The model under review builds one solid part; all positions refer to its coordinate system, in mm. A direction names the side the tool comes from. Coordinates: 2 decimals unless noted, no trailing zeros. Write each loop counter-clockwise with the first axis right and the second up, starting at its lowest first coordinate (ties: lowest second). Pieces come first, ordered by that corner, then holes. Notation, with made-up numbers: (25, 13) - (68, 13) arc R18 cw to (68, 48) - close; hole circle Ø4 at (76.5, 56). An arc over 180 degrees is marked (long way). Return JSON: item names as keys, results as strings. Group by question number.
(1) To check wall thickness, follow L1, parallel to X at y = -14, z = 0; L2, parallel to Y at x = -13, z = 0; L3, parallel to X at y = 111.5, z = -5. State the ranges of each line that lie inside material, in increasing order. Write a range as from..to.
(2) Draft analysis for pull direction Z (two halves, no side actions). For faces 5 (the face through (-11.229, 129.626, 0.21)), 6 (the face through (-128.803, -49.939, -23.115)), 7 (the face through (-15.173, 87, 14)), state which applies: released by +Z, released by -Z, zero draft, split by the parting line, or undercut.
(3) For pin 1 Ø6 at (x, z) = (-61.5, -27) entering from +Y; pin 2 Ø5 at (x, z) = (-139, -13.5) entering from +Y; pin 3 Ø12 at (x, z) = (-78.5, -12) entering from -Y; pin 4 Ø20 at (y, z) = (81.5, -4.5) entering from +X, all flat-tipped, find the tip position at first contact; note any pin that passes through.
(4) We need section A-A on y = 108. State the section outline as (x, z) points.
(5) We need section B-B on z = 0. Give the number of separate pieces and of enclosed holes in the cut face, then the cut area to 3 significant figures.
(6) Tool access review of faces 1 (the face through (-128.158, -23.317, 2.278)), 2 (the face through (-11.229, 58.59, -17.833)), 3 (the face through (-15.173, 62, 0)), 4 (the face through (-120.198, -49.939, 2.44)): name each direction out of +Z, -Z, +X, -X, +Y, -Y from which nothing blocks a thin tool from reaching the whole face with its end or side.
```python
from build123d import *

# Parameters (mm, degrees)
SWEEP1_PROFILE_R    = 21.5
BOSS_EXTRUDE1_DEPTH = 8
BOSS_EXTRUDE2_DEPTH = 8
SKETCH10_R          = 20
CUT_EXTRUDE1_DEPTH  = 8
SKETCH12_R          = 20
CUT_EXTRUDE2_DEPTH  = 8
SKETCH13_R          = 5.5
CUT_EXTRUDE3_DEPTH  = 22
SKETCH14_R          = 5.5
CUT_EXTRUDE4_DEPTH  = 22
SKETCH26_R          = 14.308639319
CUT_EXTRUDE6_DEPTH  = 75
SKETCH27_R          = 17.5
CUT_EXTRUDE8_DEPTH  = 46


with BuildPart() as part:
    # Sweep1: sweep along a path in Sketch1
    with BuildLine(Plane.XY) as sweep1_path:
        Line((-15.173427297, 84.340140469), (-59.008690724, 84.340140469))
        ThreePointArc((-59.008690724, 84.340140469), (-120.173427297, 59.004877041), (-145.508690724, -2.159859531))
        Line((-145.508690724, -2.159859531), (-145.508690724, -45.995122959))
    # Sweep1 profile (on start of the path) → Sweep1 (sweep)
    with BuildSketch(Plane(origin=(-15.173427297, 84.340140469, 0), x_dir=(0, 0, -1), z_dir=(-1, 0, 0))):
        Circle(SWEEP1_PROFILE_R)
    sweep(path=sweep1_path.line)

    # Sketch8 → Boss-Extrude1 (add)
    with BuildSketch(Plane(origin=(-15.173427297, 0, 0), x_dir=(0, 0, -1), z_dir=(1, 0, 0))):
        with BuildLine():
            Line((11.654299247, 121.647035289), (23.308607816, 91.595469986))
            ThreePointArc((23.308607816, 91.595469986), (25.000007686, 82.556156629), (23.308607816, 73.516843272))
            Line((23.308607816, 73.516843272), (12.201254362, 43.23933866))
            ThreePointArc((12.201254362, 43.23933866), (0, 34.751015799), (-12.201254362, 43.23933866))
            Line((-12.201254362, 43.23933866), (-23.308607816, 73.516843272))
            ThreePointArc((-23.308607816, 73.516843272), (-25.000007686, 82.556156629), (-23.308607816, 91.595469986))
            Line((-23.308607816, 91.595469986), (-11.654299247, 121.647035289))
            ThreePointArc((-11.654299247, 121.647035289), (0, 129.627377221), (11.654299247, 121.647035289))
        make_face()
    extrude(amount=BOSS_EXTRUDE1_DEPTH)

    # Sketch9 → Boss-Extrude2 (add)
    with BuildSketch(Plane.XZ.offset(45.995122959)):
        with BuildLine():
            Line((-157.861790456, 37.103058549), (-165.135770102, 17.103058549))
            ThreePointArc((-165.135770102, 17.103058549), (-170.186132718, 1.393320876), (-164.347898171, -14.040960373))
            Line((-164.347898171, -14.040960373), (-157.880174747, -34.040960373))
            ThreePointArc((-157.880174747, -34.040960373), (-145.361790456, -45.396941451), (-132.972897727, -33.899829272))
            Line((-132.972897727, -33.899829272), (-124.515630897, -12.02434059))
            ThreePointArc((-124.515630897, -12.02434059), (-120.202124379, 2.657801138), (-125.252486994, 17.103058549))
            Line((-125.252486994, 17.103058549), (-132.861790456, 37.103058549))
            ThreePointArc((-132.861790456, 37.103058549), (-145.361790456, 49.603058549), (-157.861790456, 37.103058549))
        make_face()
    extrude(amount=BOSS_EXTRUDE2_DEPTH)

    # Sketch10 → Cut-Extrude1 (cut)
    with BuildSketch(Plane(origin=(-7.173427297, 0, 0), x_dir=(0, 0, -1), z_dir=(1, 0, 0))):
        with Locations((0, 82.556156629)):
            Circle(SKETCH10_R)
    extrude(amount=-CUT_EXTRUDE1_DEPTH, mode=Mode.SUBTRACT)

    # Sketch12 → Cut-Extrude2 (cut)
    with BuildSketch(Plane.XZ.offset(53.995122959)):
        with Locations(Location((-145.194128548, 2.025561007, 0), (0, 0, 270))):
            Circle(SKETCH12_R)
    extrude(amount=-CUT_EXTRUDE2_DEPTH, mode=Mode.SUBTRACT)

    # Sketch13 → Cut-Extrude3 (cut)
    with BuildSketch(Plane.XZ.offset(45.995122959)):
        with Locations(Location((-145.361790456, 37.103058549, 0), (0, 0, 270))):
            Circle(SKETCH13_R)
        with Locations(Location((-145.432617565, -32.897142112, 0), (0, 0, 270))):
            Circle(SKETCH13_R)
    extrude(amount=CUT_EXTRUDE3_DEPTH, mode=Mode.SUBTRACT)

    # Sketch14 → Cut-Extrude4 (cut)
    with BuildSketch(Plane(origin=(-7.173427297, 0, 0), x_dir=(0, 0, -1), z_dir=(1, 0, 0))):
        with Locations((0, 117.127377221)):
            Circle(SKETCH14_R)
        with Locations((0, 47.764318698)):
            Circle(SKETCH14_R)
    extrude(amount=-CUT_EXTRUDE4_DEPTH, mode=Mode.SUBTRACT)

    # Sketch26 → Cut-Extrude6 (cut)
    with BuildSketch(Plane(origin=(-15.173427297, 0, 0), x_dir=(0, 0, -1), z_dir=(1, 0, 0))):
        with Locations((0, 82.556156629)):
            Circle(SKETCH26_R)
    extrude(amount=-CUT_EXTRUDE6_DEPTH, mode=Mode.SUBTRACT)

    # Sketch27 → Cut-Extrude8 (cut)
    with BuildSketch(Plane.XZ.offset(45.995122959)):
        with Locations(Location((-145.508690724, 0, 0), (0, 0, 270))):
            Circle(SKETCH27_R)
    extrude(amount=-CUT_EXTRUDE8_DEPTH, mode=Mode.SUBTRACT)


solid = part.part
```
Ans:
{
 "1": {"L1": "-167.01..-163.01, -128.01..-124.01", "L2": "34.75..42.26, 53.26..62.56, 102.56..111.63, 122.63..129.63", "L3": "-15.17..-7.17"},
 "2": {"face 5": "split by the parting line", "face 6": "released by -Z", "face 7": "undercut"},
 "3": {"pin 1": "through", "pin 2": "y = 67.17", "pin 3": "y = 59.9", "pin 4": "x = -15.17"},
 "4": {"outline": "(-15.17, -16.95) - (-7.17, -16.95) - (-7.17, 16.95) - (-15.17, 16.95) - close"},
 "5": {"separate pieces": "4", "enclosed holes": "0", "area": "6,200 mm²"},
 "6": {"face 1": "-Y", "face 2": "-Z, +X, -Y", "face 3": "none", "face 4": "+X, -Y"}
}
